from build123d import *

# Parameters (mm, degrees)
ESQUISSE1_W               = 39.4
ESQUISSE1_H               = 25.5
ESQUISSE1_R               = 1.5
ESQUISSE1_W_2             = 3
ESQUISSE1_H_2             = 8
T_LE_DE_BASE_PLI_E1_DEPTH = 3
CONG_1_R                  = 3


# Sheet-metal steps are written as plain solids
with BuildPart() as part:
    # Esquisse1 → Tôle de base pliée1 (new body)
    with BuildSketch(Plane.XY):
        with Locations((873.243101599, 1995.085790402)):
            Rectangle(ESQUISSE1_W, ESQUISSE1_H)
        with Locations((869.143101599, 2005.035790402)):
            Circle(ESQUISSE1_R, mode=Mode.SUBTRACT)
        with Locations((869.143101599, 1985.135577488)):
            Circle(ESQUISSE1_R, mode=Mode.SUBTRACT)
        Polygon((857.743101599, 1997.985790402), (855.543101599, 1997.985790402), (855.543101599, 1992.985790402), (857.743101599, 1992.985790402), (857.743101599, 1989.235790402), (880.743101599, 1989.235790402), (880.743101599, 2001.735790402), (857.743101599, 2001.735790402), align=None, mode=Mode.SUBTRACT)
        with Locations((889.243101599, 1995.635790402)):
            Rectangle(ESQUISSE1_W_2, ESQUISSE1_H_2, mode=Mode.SUBTRACT)
    extrude(amount=-T_LE_DE_BASE_PLI_E1_DEPTH)

    # Congé1
    cong_1_edges = [part.edges().sort_by_distance(p)[0] for p in [
        (853.543101599, 2007.835790402, -1.5),
        (892.943101599, 2007.835790402, -1.5),
        (892.943101599, 1982.335790402, -1.5),
        (853.543101599, 1982.335790402, -1.5),
    ]]
    fillet(cong_1_edges, radius=CONG_1_R)


solid = part.part
Build history of the part. All positions in model axes, mm. A direction names the side the tool comes from. Coordinates: 2 decimals unless noted, no trailing zeros. Write each loop counter-clockwise with the first axis right and the second up, starting at its lowest first coordinate (ties: lowest second). Pieces come first, ordered by that corner, then holes.
(1) Drill centre lines: line 1 (X direction, y = 1991.75, z = -1.25); line 2 (X direction, y = 1994, z = -1.7); line 3 (X direction, y = 2000.75, z = -0.15). Where is each one in solid material? Low to high.
(2) Cut at B-B on y = 1993.75. List the corners of the cut face in (x, z), and give its area (3 significant figures).
(3) Mould opens along X. For faces 1 (the flat face through (873, 1982.336, -1)), 2 (the flat face through (889, 1991.636, -1)), 3 (the cylindrical face through (892.04, 1983.19, -1.52)) say: pulls with the +X half, pulls with the -X half, needs draft (parallel to the pull), parting line crosses it, or undercut.
(4) 3-axis set-ups, long thin cutter, end or side, ignore diameter. For faces 4 (the flat face through (873, 2007.836, -1)), 5 (the flat face through (880.743, 1995, -1)): which of +Z, -Z, +X, -X, +Y, -Y reach the whole face in a straight line?
(5) Cut at A-A on x = 872. List the corners of the cut face in (y, z), and give its area (3 significant figures).
(6) Cut at D-D on z = -1.4. List the corners of the cut face in (x, y).
(7) Cut at C-C on y = 1990. List the corners of the cut face in (x, z), and give its area (3 significant figures).
Working result:
1. line 1: x = 853.54 to 857.74, 880.74 to 887.74, 890.74 to 892.94
1. line 2: x = 853.54 to 855.54, 880.74 to 887.74, 890.74 to 892.94
1. line 3: x = 853.54 to 857.74, 880.74 to 892.94
2. outline: (853.54, -3) - (855.54, -3) - (855.54, 0) - (853.54, 0) - close; (880.74, -3) - (887.74, -3) - (887.74, 0) - (880.74, 0) - close; (890.74, -3) - (892.94, -3) - (892.94, 0) - (890.74, 0) - close
2. area: 33.6 mm2
3. face 1: needs draft
3. face 2: undercut
3. face 3: pulls with the +X half
4. face 4: +Z, -Z, +X, -X, +Y
4. face 5: +Z, -Z
5. outline: (1982.34, -3) - (1989.24, -3) - (1989.24, 0) - (1982.34, 0) - close; (2001.74, -3) - (2007.84, -3) - (2007.84, 0) - (2001.74, 0) - close
5. area: 39.0 mm2
6. outline: (853.54, 1985.34) arc R3 ccw to (856.54, 1982.34) - (889.94, 1982.34) arc R3 ccw to (892.94, 1985.34) - (892.94, 2004.84) arc R3 ccw to (889.94, 2007.84) - (856.54, 2007.84) arc R3 ccw to (853.54, 2004.84) - close; hole (855.54, 1992.99) - (857.74, 1992.99) - (857.74, 1989.24) - (880.74, 1989.24) - (880.74, 2001.74) - (857.74, 2001.74) - (857.74, 1997.99) - (855.54, 1997.99) - close; hole circle Ø3 at (869.14, 1985.14); hole circle Ø3 at (869.14, 2005.04); hole (887.74, 1991.64) - (890.74, 1991.64) - (890.74, 1999.64) - (887.74, 1999.64) - close
7. outline: (853.54, -3) - (857.74, -3) - (857.74, 0) - (853.54, 0) - close; (880.74, -3) - (892.94, -3) - (892.94, 0) - (880.74, 0) - close
7. area: 49.2 mm2
